Source: CAD feature listing. Evaluate the final solid. Frame: model axes, mm. A direction names the side the tool comes from. Coordinates: 2 decimals unless noted, no trailing zeros. Order: outer loops, then holes, each group sorted by start corner. A loop starts at its lowest first (then second) coordinate and runs counter-clockwise, first axis right, second up. Notation, with made-up numbers: (-7.75, 30) -> (38.25, 30) arc R9 ccw to (38.25, 40) -> close; hole circle Ø6 at (59.5, 78.25). An arc over 180 degrees is marked (long way). Write item = value, one per line. Start each with the question number.
Item 1: Ray query, line 1 along Y through (x, z) = (30, -0.8); line 2 along Z through (x, y) = (46.5, 4.5); line 3 along Y through (x, z) = (7.5, 3). Return the intervals inside material, ascending. Write a range as [from, to].
Item 2: Mould query, pull axis X, two halves, no side actions, for faces 1 (the cylindrical face through (3.487, 0.972, 42.85)), 2 (the flat face through (35, 8, -1)), 3 (the cylindrical face through (47.361, 5.427, -2.857)), 4 (the flat face through (22, 5, -1)). Classes: released by +X, released by -X, zero draft, split by the parting line, or undercut.
Item 3: Section query B-B (z = 6). Output: boundary loops of the cut face in (x, y).
Item 4: Set-up query: faces 5 (the flat face through (30, 4, -1.8)), 6 (the flat face through (35, 2, -3)), 7 (the flat face through (4, 3, 17)). Return all of +Z, -Z, +X, -X, +Y, -Y with unobstructed straight access to the full face (end or side cutting, diameter ignored); none if empty.
Item 5: Section query D-D (x = 18). Output: boundary loops of the cut face in (y, z).
Item 6: Section query C-C (x = 26). Output: boundary loops of the cut face in (y, z), then the cut area to 3 significant figures.
Item 7: Section query A-A (x = 40). Output: boundary loops of the cut face in (y, z), then the cut area to 3 significant figures.
Item 8: Contact query for flat-ended pins moving along their axis: pin 1 (1.5 mm diameter, centred on x = 12.5, z = 18, fed in from +Y); pin 2 (9.5 mm diameter, centred on x = 6.5, z = 27.5, fed in from +Y); pin 3 (4 mm diameter, centred on y = 6, z = 9.5, fed in from +X); pin 4 (4.5 mm diameter, centred on x = 29.5, y = 3.5, fed in from +Z). Output: stop coordinate, or through.
```python
from build123d import *

# Parameters (mm, degrees)
BOSS_EXTRUDE1_DEPTH = 43
SKETCH1_3_R         = 2.15
BOSS_EXTRUDE2_DEPTH = 3
SKETCH1_5_R         = 2.15
CUT_EXTRUDE1_DEPTH  = 1.8
FILLET1_R           = 0.5


with BuildPart() as part:
    # Sketch1 → Boss-Extrude1 (new body)
    with BuildSketch(Plane.XY):
        Polygon((2.717157288, 0), (3, 0), (35, 0), (35, -2), (0, -2), (0, 3), (4.8, 3), (4.8, 2.082842712), (2.858578644, 0.141421356), align=None)
    extrude(amount=BOSS_EXTRUDE1_DEPTH)

    # Sketch1_3 → Boss-Extrude2 (add)
    # profile 1 of 3: a face of its own
    with BuildSketch(Plane.XY):
        Polygon((2.717157288, 0), (3, 0), (35, 0), (35, -2), (0, -2), (0, 3), (4.8, 3), (4.8, 2.082842712), (2.858578644, 0.141421356), align=None)
    # profile 2 of 3: a face of its own
    with BuildSketch(Plane.XY):
        Polygon((35, 8), (35, 3), (35, 0), (3, 0), (2.717157288, 0), (2.858578644, 0.141421356), (4.8, 2.082842712), (4.8, 3), (20, 3), (25, 8), align=None)
        with Locations((30, 4)):
            Circle(SKETCH1_3_R, mode=Mode.SUBTRACT)
    # profile 3 of 3: a face of its own
    with BuildSketch(Plane.XY):
        with Locations((30, 4)):
            Circle(SKETCH1_3_R)
    extrude(amount=-BOSS_EXTRUDE2_DEPTH)

    # Sketch1_5 → Cut-Extrude1 (cut)
    with BuildSketch(Plane.XY):
        with Locations((30, 4)):
            Circle(SKETCH1_5_R)
    extrude(amount=-CUT_EXTRUDE1_DEPTH, mode=Mode.SUBTRACT)

    # Mirror1: part across plane


with BuildPart() as part_1:
    add(part.part)
    add(part.part.mirror(Plane(origin=(35, 0, 43), x_dir=(0, 0, 1), z_dir=(-1, 0, 0))))

    # Fillet1
    fillet1_edges = [part_1.edges().sort_by_distance(p)[0] for p in [
        (3.758578644, 1.041421356, 43),
        (0, -2, 20),
        (0, 3, 20),
        (4.8, 3, 21.5),
        (4.8, 2.082842712, 21.5),
        (4.8, 2.541421356, 43),
        (2.4, 3, 43),
        (12.4, 3, 0),
        (0, 0.5, 43),
        (22.5, 5.5, 0),
        (20, 3, -1.5),
        (35, 8, 0),
        (25, 8, -1.5),
        (35, -2, -3),
        (0, 0.5, -3),
        (10, 3, -3),
        (22.5, 5.5, -3),
        (35, 8, -3),
        (35, -2, 43),
        (27.85, 4, 0),
        (65.2, 2.082842712, 21.5),
        (65.2, 3, 21.5),
        (70, 3, 20),
        (60, 3, -3),
        (50, 3, -1.5),
        (70, -2, 20),
        (70, 0.5, -3),
        (35, 0, 43),
        (70, 0.5, 43),
        (67.6, 3, 43),
        (65.2, 2.541421356, 43),
        (66.241421356, 1.041421356, 43),
        (47.5, 5.5, -3),
        (45, 8, -1.5),
        (42.15, 4, 0),
        (57.6, 3, 0),
        (47.5, 5.5, 0),
    ]]
    fillet(fillet1_edges, radius=FILLET1_R)


solid = part_1.part
```
Computed:
q1.line_1 = [-2, 1.85], [6.15, 8]
q1.line_2 = [-3, 0]
q1.line_3 = [-2, 0]
q2.face_1 = undercut
q2.face_2 = zero draft
q2.face_3 = released by +X
q2.face_4 = released by -X
q3.outline = (0, -1.5) arc R0.5 ccw to (0.5, -2) -> (69.5, -2) arc R0.5 ccw to (70, -1.5) -> (70, 2.5) arc R0.5 ccw to (69.5, 3) -> (65.7, 3) arc R0.5 ccw to (65.2, 2.5) -> (65.2, 2.29) arc R0.5 ccw to (65.35, 1.94) -> (67.28, 0) -> (2.72, 0) -> (4.65, 1.94) arc R0.5 ccw to (4.8, 2.29) -> (4.8, 2.5) arc R0.5 ccw to (4.3, 3) -> (0.5, 3) arc R0.5 ccw to (0, 2.5) -> close
q4.face_5 = +Z
q4.face_6 = -Z, +X, -X, +Y, -Y
q4.face_7 = +Z, -Z, -X, +Y
q5.outline = (-2, -2.5) arc R0.5 ccw to (-1.5, -3) -> (2.5, -3) arc R0.5 ccw to (3, -2.5) -> (3, -0.5) arc R0.5 ccw to (2.5, 0) -> (0, 0) -> (0, 42.5) arc R0.5 ccw to (-0.5, 43) -> (-1.5, 43) arc R0.5 ccw to (-2, 42.5) -> close
q6.outline = (-2, -2.5) arc R0.5 ccw to (-1.5, -3) -> (7.5, -3) arc R0.5 ccw to (8, -2.5) -> (8, -0.5) arc R0.5 ccw to (7.5, 0) -> (0, 0) -> (0, 42.5) arc R0.5 ccw to (-0.5, 43) -> (-1.5, 43) arc R0.5 ccw to (-2, 42.5) -> close
q6.area = 116 mm^2
q7.outline = (-2, -2.5) arc R0.5 ccw to (-1.5, -3) -> (7.5, -3) arc R0.5 ccw to (8, -2.5) -> (8, -0.5) arc R0.5 ccw to (7.5, 0) -> (6.65, 0) arc R0.5 ccw to (6.15, -0.5) -> (6.15, -1.8) -> (1.85, -1.8) -> (1.85, -0.5) arc R0.5 ccw to (1.35, 0) -> (0, 0) -> (0, 42.5) arc R0.5 ccw to (-0.5, 43) -> (-1.5, 43) arc R0.5 ccw to (-2, 42.5) -> close
q7.area = 108 mm^2
q8.pin_1 = 0
q8.pin_2 = 3
q8.pin_3 = through
q8.pin_4 = 0
